from build123d import *

# Parameters (mm, degrees)
F0_W     = 304.8
F0_H     = 304.8
F1_DEPTH = 152.4
F2_W     = 152.4
F2_H     = 152.4
F3_DEPTH = 304.801
F4_W     = 152.4
F4_H     = 152.4
F5_DEPTH = 304.801
F6_W     = 152.4
F6_H     = 152.4
F7_DEPTH = 304.801


with BuildPart() as f1:
    # F0 (on Front) → F1 (new body, symmetric)
    with BuildSketch(Plane.XZ):
        Rectangle(F0_W, F0_H)
    extrude(amount=F1_DEPTH, both=True)

    # F2 (on face) → F3 (cut, through all)
    with BuildSketch(Plane.YZ.offset(152.4)):
        Rectangle(F2_W, F2_H)
    extrude(amount=-F3_DEPTH, mode=Mode.SUBTRACT)

    # F4 (on face) → F5 (cut, through all)
    with BuildSketch(Plane.XZ.offset(152.4)):
        Rectangle(F4_W, F4_H)
    extrude(amount=-F5_DEPTH, mode=Mode.SUBTRACT)

    # F6 (on face) → F7 (cut, through all)
    with BuildSketch(Plane.XY.offset(152.4)):
        Rectangle(F6_W, F6_H)
    extrude(amount=-F7_DEPTH, mode=Mode.SUBTRACT)


solid = f1.part
Model file for the job. Use its own axes, mm. A direction names the side the tool comes from. Coordinates: 2 decimals unless noted, no trailing zeros. Write each loop counter-clockwise with the first axis right and the second up, starting at its lowest first coordinate (ties: lowest second). Pieces come first, ordered by that corner, then holes. Notation, with made-up numbers: (35, 45) -> (89, 45) arc R32 cw to (89, 80) -> close; hole circle Ø5 at (-6, 6). An arc over 180 degrees is marked (long way). One line per item, written item: value. Start each with the question number.
1) Which spindle directions (+Z, -Z, +X, -X, +Y, -Y) get a long thin tool onto all of the face, cutting with end or side? Do faces 1 (the face through (-76.2, -115, -1)), 2 (the face through (115, -76.2, -1)), 3 (the face through (-1, 76.2, 115)). Say none if no direction does.
2) Slice it at A-A on y = -49.5. Write the cut outline in (x, z), then the cut area to 3 significant figures.
3) Slice it at C-C on x = 99.5. Write the cut outline in (y, z).
4) Probe probe 1 along X at (y, z) = (130, 72.5). List the from-to ranges inside material, lowest first.
5) Pull direction Z, two halves, no side cores. Call faces 4 (the face through (-114, -1, -76.2)), 5 (the face through (76.2, -1, 115)), 6 (the face through (-2, -104, -152.4)): +Z half, -Z half, draft (parallel to the pull), parting line (faces both ways), or undercut.
Answers follow:
1. face 1: +Y, -Y
1. face 2: +X, -X
1. face 3: +Z, -Z
2. outline: (-152.4, -152.4) -> (-76.2, -152.4) -> (-76.2, -76.2) -> (-152.4, -76.2) -> close; (-152.4, 76.2) -> (-76.2, 76.2) -> (-76.2, 152.4) -> (-152.4, 152.4) -> close; (76.2, -152.4) -> (152.4, -152.4) -> (152.4, -76.2) -> (76.2, -76.2) -> close; (76.2, 76.2) -> (152.4, 76.2) -> (152.4, 152.4) -> (76.2, 152.4) -> close
2. area: 23,200 mm2
3. outline: (-152.4, -152.4) -> (152.4, -152.4) -> (152.4, 152.4) -> (-152.4, 152.4) -> close; hole (-76.2, -76.2) -> (76.2, -76.2) -> (76.2, 76.2) -> (-76.2, 76.2) -> close
4. probe 1: -152.4 to -76.2, 76.2 to 152.4
5. face 4: undercut
5. face 5: draft
5. face 6: -Z half
